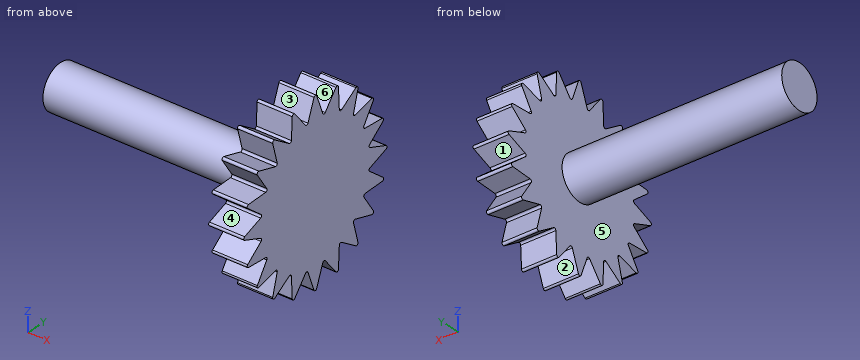
```python
from build123d import *

# Parameters (mm, degrees)
F1_DEPTH = 4
F2_R     = 2.5
F3_DEPTH = 25


with BuildPart() as f1:
    # F0 (on Right) → F1 (new body)
    with BuildSketch(Plane.YZ):
        with BuildLine():
            ThreePointArc((0.186993, 10.007145), (0, 10.136198), (-0.186993, 10.007145))
            Line((-0.186993, 10.007145), (-1.049264, 7.734473))
            ThreePointArc((-1.049264, 7.734473), (-1.20497, 7.607883), (-1.392175, 7.680162))
            Line((-1.392175, 7.680162), (-2.914536, 9.575144))
            ThreePointArc((-2.914536, 9.575144), (-3.132257, 9.640097), (-3.270219, 9.459576))
            Line((-3.270219, 9.459576), (-3.387993, 7.031681))
            ThreePointArc((-3.387993, 7.031681), (-3.49696, 6.86317), (-3.697337, 6.874062))
            Line((-3.697337, 6.874062), (-5.730771, 8.205862))
            ThreePointArc((-5.730771, 8.205862), (-5.957908, 8.200356), (-6.033333, 7.986038))
            Line((-6.033333, 7.986038), (-5.395082, 5.640579))
            ThreePointArc((-5.395082, 5.640579), (-5.446643, 5.446643), (-5.640579, 5.395082))
            Line((-5.640579, 5.395082), (-7.986038, 6.033333))
            ThreePointArc((-7.986038, 6.033333), (-8.200356, 5.957908), (-8.205862, 5.730771))
            Line((-8.205862, 5.730771), (-6.874062, 3.697337))
            ThreePointArc((-6.874062, 3.697337), (-6.86317, 3.49696), (-7.031681, 3.387993))
            Line((-7.031681, 3.387993), (-9.459576, 3.270219))
            ThreePointArc((-9.459576, 3.270219), (-9.640097, 3.132257), (-9.575144, 2.914536))
            Line((-9.575144, 2.914536), (-7.680162, 1.392175))
            ThreePointArc((-7.680162, 1.392175), (-7.607883, 1.20497), (-7.734473, 1.049264))
            Line((-7.734473, 1.049264), (-10.007145, 0.186993))
            ThreePointArc((-10.007145, 0.186993), (-10.136198, 0), (-10.007145, -0.186993))
            Line((-10.007145, -0.186993), (-7.734473, -1.049264))
            ThreePointArc((-7.734473, -1.049264), (-7.607883, -1.20497), (-7.680162, -1.392175))
            Line((-7.680162, -1.392175), (-9.575144, -2.914536))
            ThreePointArc((-9.575144, -2.914536), (-9.640097, -3.132257), (-9.459576, -3.270219))
            Line((-9.459576, -3.270219), (-7.031681, -3.387993))
            ThreePointArc((-7.031681, -3.387993), (-6.86317, -3.49696), (-6.874062, -3.697337))
            Line((-6.874062, -3.697337), (-8.205862, -5.730771))
            ThreePointArc((-8.205862, -5.730771), (-8.200356, -5.957908), (-7.986038, -6.033333))
            Line((-7.986038, -6.033333), (-5.640579, -5.395082))
            ThreePointArc((-5.640579, -5.395082), (-5.446643, -5.446643), (-5.395082, -5.640579))
            Line((-5.395082, -5.640579), (-6.033333, -7.986038))
            ThreePointArc((-6.033333, -7.986038), (-5.957908, -8.200356), (-5.730771, -8.205862))
            Line((-5.730771, -8.205862), (-3.697337, -6.874062))
            ThreePointArc((-3.697337, -6.874062), (-3.49696, -6.86317), (-3.387993, -7.031681))
            Line((-3.387993, -7.031681), (-3.270219, -9.459576))
            ThreePointArc((-3.270219, -9.459576), (-3.132257, -9.640097), (-2.914536, -9.575144))
            Line((-2.914536, -9.575144), (-1.392175, -7.680162))
            ThreePointArc((-1.392175, -7.680162), (-1.20497, -7.607883), (-1.049264, -7.734473))
            Line((-1.049264, -7.734473), (-0.186993, -10.007145))
            ThreePointArc((-0.186993, -10.007145), (0, -10.136198), (0.186993, -10.007145))
            Line((0.186993, -10.007145), (1.049264, -7.734473))
            ThreePointArc((1.049264, -7.734473), (1.20497, -7.607883), (1.392175, -7.680162))
            Line((1.392175, -7.680162), (2.914536, -9.575144))
            ThreePointArc((2.914536, -9.575144), (3.132257, -9.640097), (3.270219, -9.459576))
            Line((3.270219, -9.459576), (3.387993, -7.031681))
            ThreePointArc((3.387993, -7.031681), (3.49696, -6.86317), (3.697337, -6.874062))
            Line((3.697337, -6.874062), (5.730771, -8.205862))
            ThreePointArc((5.730771, -8.205862), (5.957908, -8.200356), (6.033333, -7.986038))
            Line((6.033333, -7.986038), (5.395082, -5.640579))
            ThreePointArc((5.395082, -5.640579), (5.446643, -5.446643), (5.640579, -5.395082))
            Line((5.640579, -5.395082), (7.986038, -6.033333))
            ThreePointArc((7.986038, -6.033333), (8.200356, -5.957908), (8.205862, -5.730771))
            Line((8.205862, -5.730771), (6.874062, -3.697337))
            ThreePointArc((6.874062, -3.697337), (6.86317, -3.49696), (7.031681, -3.387993))
            Line((7.031681, -3.387993), (9.459576, -3.270219))
            ThreePointArc((9.459576, -3.270219), (9.640097, -3.132257), (9.575144, -2.914536))
            Line((9.575144, -2.914536), (7.680162, -1.392175))
            ThreePointArc((7.680162, -1.392175), (7.607883, -1.20497), (7.734473, -1.049264))
            Line((7.734473, -1.049264), (10.007145, -0.186993))
            ThreePointArc((10.007145, -0.186993), (10.136198, 0), (10.007145, 0.186993))
            Line((10.007145, 0.186993), (7.734473, 1.049264))
            ThreePointArc((7.734473, 1.049264), (7.607883, 1.20497), (7.680162, 1.392175))
            Line((7.680162, 1.392175), (9.575144, 2.914536))
            ThreePointArc((9.575144, 2.914536), (9.640097, 3.132257), (9.459576, 3.270219))
            Line((9.459576, 3.270219), (7.031681, 3.387993))
            ThreePointArc((7.031681, 3.387993), (6.86317, 3.49696), (6.874062, 3.697337))
            Line((6.874062, 3.697337), (8.205862, 5.730771))
            ThreePointArc((8.205862, 5.730771), (8.200356, 5.957908), (7.986038, 6.033333))
            Line((7.986038, 6.033333), (5.640579, 5.395082))
            ThreePointArc((5.640579, 5.395082), (5.446643, 5.446643), (5.395082, 5.640579))
            Line((5.395082, 5.640579), (6.033333, 7.986038))
            ThreePointArc((6.033333, 7.986038), (5.957908, 8.200356), (5.730771, 8.205862))
            Line((5.730771, 8.205862), (3.697337, 6.874062))
            ThreePointArc((3.697337, 6.874062), (3.49696, 6.86317), (3.387993, 7.031681))
            Line((3.387993, 7.031681), (3.270219, 9.459576))
            ThreePointArc((3.270219, 9.459576), (3.132257, 9.640097), (2.914536, 9.575144))
            Line((2.914536, 9.575144), (1.392175, 7.680162))
            ThreePointArc((1.392175, 7.680162), (1.20497, 7.607883), (1.049264, 7.734473))
            Line((1.049264, 7.734473), (0.186993, 10.007145))
        make_face()
    extrude(amount=F1_DEPTH)

    # F2 (on Right) → F3 (join)
    with BuildSketch(Plane.YZ):
        Circle(F2_R)
    extrude(amount=-F3_DEPTH)


solid = f1.part
```
The model under review builds one solid part; all positions refer to its coordinate system, in mm. Face numbers are marked on the shaded views. A direction names the side the tool comes from. Round coordinates to 2 decimals unless told otherwise and drop trailing zeros. Loops run counter-clockwise (first coordinate to the right, second up) from the corner with the lowest first, then second, coordinate; pieces in that order, holes last. Notation, with made-up numbers: (54.5, 77.5) - (84.5, 77.5) arc R23 ccw to (84.5, 109.5) - close; hole circle Ø8 at (84, -23). An arc over 180 degrees is marked (long way). Use a Markdown table: item, result. Add a question column.
Q1. Add section A-A (y = -4.75). State the section outline as (x, z) points.
Q2. For probe 1 along Z at (x, y) = (2.25, 7); probe 2 along X at (y, z) = (3.25, -8); probe 3 along Y at (x, z) = (-1, 1.5), list the stretches that pass through material, from the lowest coordinate up.
Q3. Insertion check: pin 1 Ø5 at (x, z) = (-15.5, 1.5) entering from +Y; pin 2 Ø1.5 at (x, y) = (-12, -1.5) entering from -Z; pin 3 Ø10 at (x, z) = (-8, 3) entering from -Y. Each pin has a flat end and moves straight along its axis. Give the tip position at first contact, or say it passes through.
Q4. Add section B-B (x = -15). State the section outline as (y, z) points.
Q5. The part is to be moulded in two halves that separate along Y. For the marked faces 4, 5 and 6, say which applies: pulls with the +Y half, pulls with the -Y half, needs draft (parallel to the pull), parting line crosses it, or undercut.
Q6. Machinability: for the marked faces 1, 2 and 3, which of the approach directions +Z, -Z, +X, -X, +Y, -Y give a long, thin tool a straight path to every point of the face, cutting with its end or side? Answer none if there is none.
Worked answers:
| question | item | result |
|---|---|---|
| 1 | outline | (0, -7.56) - (4, -7.56) - (4, 7.56) - (0, 7.56) - close |
| 2 | probe 1 | -5.77 to -3.89, -3.39 to 3.39, 3.89 to 5.77 |
| 2 | probe 2 | 0 to 4 |
| 2 | probe 3 | -2 to 2 |
| 3 | pin 1 | y = 2.5 |
| 3 | pin 2 | z = -2.38 |
| 3 | pin 3 | y = -2.5 |
| 4 | outline | circle Ø5 at (0, 0) |
| 5 | face 4 | pulls with the -Y half |
| 5 | face 5 | needs draft |
| 5 | face 6 | undercut |
| 6 | face 1 | +X, -X, +Y |
| 6 | face 2 | -Z, +X, -X |
| 6 | face 3 | +Z, +X, -X |
